Can you work these out from the model? Positions are in its coordinate system, mm. Face numbers are marked on the shaded views. A direction names the side the tool comes from. Coordinates: 2 decimals unless noted, no trailing zeros. Order: outer loops, then holes, each group sorted by start corner. A loop starts at its lowest first (then second) coordinate and runs counter-clockwise, first axis right, second up. Notation, with made-up numbers: (51.5, -3.75) -> (92.5, -3.75) arc R25 ccw to (92.5, 29.25) -> close; hole circle Ø2 at (61.25, -26). An arc over 180 degrees is marked (long way). Answer in a Markdown table with one row per item. Add a question column.
1. Will these pins go through, and if not, where does the flat tip stop? pin 1 (1.8 mm diameter, centred on x = 30, y = 5.5, fed in from -Z); pin 2 (4.5 mm diameter, centred on x = 3, y = 4, fed in from -Z); pin 3 (10 mm diameter, centred on x = 27.5, y = 13, fed in from +Z).
2. Imagine slicing it at A-A on z = -22.95. Write out the boundary of the cut face in (x, y), plus the area to 4 significant figures.
3. Imagine slicing it at B-B on y = 2.25. Write out the boundary of the cut face in (x, z), plus the area to 3 significant figures.
4. We'd pull the mould along X, two halves only. Please class the marked faces 1, 2, 3 and 4: pulls with the +X half, pulls with the -X half, needs draft (parallel to the pull), parting line crosses it, or undercut.
5. Imagine slicing it at C-C on z = -18. Write out the boundary of the cut face in (x, y), plus the area to 3 significant figures.
6. Imagine slicing it at D-D on x = 19.5. Write out the boundary of the cut face in (y, z), plus the area to 3 significant figures.
7. If I drill on line 1 along X through (y, z) = (0.75, -22.95); line 2 along X through (y, z) = (9.5, -6.5); line 3 along Y through (x, z) = (18.5, -20), over which ranges is the centre line in solid material (lowest first)? Write a range as [from, to].
8. On a 3-axis mill with a long thin cutter (end or side, diameter ignored), from which of +Z, -Z, +X, -X, +Y, -Y can I reach the whole of each face in a straight line? I mean the marked faces 5, 6, 7, 8 and 9. Say none if no direction works.
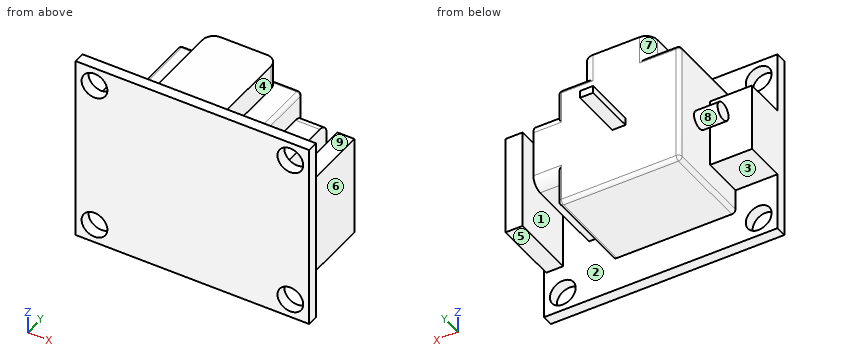
from build123d import *

# Parameters (mm, degrees)
SKETCH1_W                       = 31.7
SKETCH1_H                       = 25.5
BOSS_EXTRUDE1_DEPTH             = 1.5
F_3_0MM_DOWEL_HOLE1_D           = 3.5
F_3_0MM_DOWEL_HOLE1_ON_FACE_2_D = 3.5
BOSS_EXTRUDE2_DEPTH             = 12.2
SKETCH5_W                       = 2.3
SKETCH5_H                       = 13.7
BOSS_EXTRUDE3_DEPTH             = 8.9
SKETCH6_W                       = 5.7
SKETCH6_H                       = 9.3
BOSS_EXTRUDE4_DEPTH             = 5.6
SKETCH7_R                       = 1.2
BOSS_EXTRUDE5_DEPTH             = 3.2
FILLET2_R                       = 1.5
FILLET1_R                       = 0.5
SKETCH8_W                       = 1.8
SKETCH8_H                       = 1
BOSS_EXTRUDE6_DEPTH             = 7.1


with BuildPart() as part:
    # Sketch1 → Boss-Extrude1 (new body)
    with BuildSketch(Plane(origin=(0, 0, 0), x_dir=(1, 0, 0), z_dir=(0, 1, 0))):
        with Locations((15.85, 12.75)):
            Rectangle(SKETCH1_W, SKETCH1_H)
    extrude(amount=BOSS_EXTRUDE1_DEPTH)

    # Ø3.0mm Dowel Hole1 (through all)
    with Locations(Plane(origin=(2.55, 1.5, -22.95), x_dir=(0, 0, 1), z_dir=(0, 1, 0))):
        with Locations((0, 0), (0, 26.6), (20.4, 26.6), (20.4, 0)):
            Hole(F_3_0MM_DOWEL_HOLE1_D / 2)

    # Ø3.0mm Dowel Hole1 on face 2 (through all)
    with Locations(Plane(origin=(39.661564938, 0, -26.520963617), x_dir=(0, 0, 1), z_dir=(0, 1, 0))):
        with Locations((0, 0)):
            Hole(F_3_0MM_DOWEL_HOLE1_ON_FACE_2_D / 2)

    # Sketch4 → Boss-Extrude2 (add)
    with BuildSketch(Plane(origin=(0, 1.5, 0), x_dir=(1, 0, 0), z_dir=(0, 1, 0))):
        Polygon((5.7, 20.9), (22.3, 20.9), (22.3, 16.9), (25.6, 16.9), (25.6, 7.6), (22.3, 7.6), (22.3, 4.3), (19, 4.3), (19, 1), (9.7, 1), (9.7, 4.3), (5.7, 4.3), align=None)
    extrude(amount=BOSS_EXTRUDE2_DEPTH)

    # Sketch5 → Boss-Extrude3 (add)
    with BuildSketch(Plane(origin=(0, 1.5, 0), x_dir=(1, 0, 0), z_dir=(0, 1, 0))):
        with Locations((30.25, 12.25)):
            Rectangle(SKETCH5_W, SKETCH5_H)
    extrude(amount=BOSS_EXTRUDE3_DEPTH)

    # Sketch6 → Boss-Extrude4 (add)
    with BuildSketch(Plane(origin=(0, 1.5, 0), x_dir=(1, 0, 0), z_dir=(0, 1, 0))):
        with Locations((2.85, 12.95)):
            Rectangle(SKETCH6_W, SKETCH6_H)
    extrude(amount=BOSS_EXTRUDE4_DEPTH)

    # Sketch7 → Boss-Extrude5 (add)
    with BuildSketch(Plane.ZY.offset(-5.7)):
        with Locations(Location((-12.6, 9.4, 0), (0, 0, 180))):
            Circle(SKETCH7_R)
    extrude(amount=BOSS_EXTRUDE5_DEPTH)

    # Fillet2
    fillet2_edges = [part.edges().sort_by_distance(p)[0] for p in [
        (9.7, 13.7, -2.65),
        (19, 13.7, -2.65),
        (23.95, 13.7, -7.6),
        (23.95, 13.7, -16.9),
    ]]
    fillet(fillet2_edges, radius=FILLET2_R)

    # Fillet1
    fillet1_edges = [part.edges().sort_by_distance(p)[0] for p in [
        (5.7, 7.6, -20.9),
        (5.7, 7.6, -4.3),
        (22.3, 7.6, -4.3),
        (22.3, 7.6, -20.9),
        (5.7, 13.7, -12.6),
        (8.45, 13.7, -4.3),
        (19.9, 13.7, -4.3),
        (22.3, 13.7, -6.7),
        (22.3, 13.7, -18.15),
        (14, 13.7, -20.9),
    ]]
    fillet(fillet1_edges, radius=FILLET1_R)

    # Sketch8 → Boss-Extrude6 (add)
    with BuildSketch(Plane(origin=(0, 13.7, 0), x_dir=(1, 0, 0), z_dir=(0, 1, 0))):
        with Locations((13.991138348, 12.593671102)):
            Rectangle(SKETCH8_W, SKETCH8_H)
    extrude(amount=BOSS_EXTRUDE6_DEPTH)


solid = part.part
Answers follow:
| question | item | result |
|---|---|---|
| 1 | pin 1 | stops at z = -19.1 |
| 1 | pin 2 | stops at z = -17.6 |
| 1 | pin 3 | stops at z = -5.4 |
| 2 | outline | (0, 0) -> (0.8, 0) -> (0.8, 1.5) -> (0, 1.5) -> close; (4.3, 0) -> (27.4, 0) -> (27.4, 1.5) -> (4.3, 1.5) -> close; (30.9, 0) -> (31.7, 0) -> (31.7, 1.5) -> (30.9, 1.5) -> close |
| 2 | area | 37.05 mm² |
| 3 | outline | (0, -17.6) -> (5.7, -17.6) -> (5.7, -20.4) arc R0.5 ccw to (6.2, -20.9) -> (21.8, -20.9) arc R0.5 ccw to (22.3, -20.4) -> (22.3, -16.9) -> (25.6, -16.9) -> (25.6, -7.6) -> (22.3, -7.6) -> (22.3, -4.8) arc R0.5 ccw to (21.8, -4.3) -> (19, -4.3) -> (19, -1) -> (9.7, -1) -> (9.7, -4.3) -> (6.2, -4.3) arc R0.5 ccw to (5.7, -4.8) -> (5.7, -8.3) -> (0, -8.3) -> close; (29.1, -19.1) -> (31.4, -19.1) -> (31.4, -5.4) -> (29.1, -5.4) -> close |
| 3 | area | 421 mm² |
| 4 | face 1 | undercut |
| 4 | face 2 | undercut |
| 4 | face 3 | needs draft |
| 4 | face 4 | pulls with the +X half |
| 5 | outline | (0, 0) -> (31.7, 0) -> (31.7, 1.5) -> (31.4, 1.5) -> (31.4, 10.4) -> (29.1, 10.4) -> (29.1, 1.5) -> (22.3, 1.5) -> (22.3, 13.2) arc R0.5 ccw to (21.8, 13.7) -> (6.2, 13.7) arc R0.5 ccw to (5.7, 13.2) -> (5.7, 1.5) -> (0, 1.5) -> close |
| 5 | area | 270 mm² |
| 6 | outline | (0, -25.5) -> (1.5, -25.5) -> (1.5, -20.9) -> (13.2, -20.9) arc R0.5 ccw to (13.7, -20.4) -> (13.7, -4.8) arc R0.5 ccw to (13.2, -4.3) -> (1.5, -4.3) -> (1.5, 0) -> (0, 0) -> close |
| 6 | area | 241 mm² |
| 7 | line 1 | x = [0, 0.8], [4.3, 27.4], [30.9, 31.7] |
| 7 | line 2 | x = [5.7, 22.3], [29.1, 31.4] |
| 7 | line 3 | y = [0, 13.7] |
| 8 | face 5 | -Z, +X, +Y |
| 8 | face 6 | +Z, -Z, +X, +Y |
| 8 | face 7 | +Z, -X, +Y |
| 8 | face 8 | -X |
| 8 | face 9 | +Z, +X, +Y |
